Geometry check sheet. Reference: the model listing, model coordinates, mm. A direction names the side the tool comes from. Give positions to 0.01 mm unless a question says otherwise; leave off trailing zeros. Loops run counter-clockwise (first coordinate to the right, second up) from the corner with the lowest first, then second, coordinate; pieces in that order, holes last. Notation, with made-up numbers: (52, -37) -> (110, -37) arc R25 ccw to (110, -14) -> close; hole circle Ø11 at (7, 17.25). An arc over 180 degrees is marked (long way). Answer in a Markdown table with one row per item. Add a question column.
Autodesk Inventor part; units mm, degrees
ref_plane "YZ Plane" through (0, 0, 0) normal (1, 0, 0) x (0, 1, 0)
ref_plane "XZ Plane" through (0, 0, 0) normal (0, 1, 0) x (-1, 0, 0)
ref_plane "XY Plane" through (0, 0, 0) normal (0, 0, 1) x (1, 0, 0)
sketch "スケッチ1" plane through (0, 0, 0) normal (0, 0, 1) x (1, 0, 0)
  circle A0 centre (0, 0) radius 10
  circle A1 centre (0, 0) radius 2
  line L0 (0, -2) -> (0, -47)
  line L1 (10, 0) -> (10, -47)
  line L2 (10, -47) -> (-10, -47)
  line L3 (-10, -47) -> (-10, 0)
  circle A2 centre (0, -32) radius 1
  circle A3 centre (0, -42) radius 1
  circle A4 centre (0, -22) radius 1
  dimension "d1" = 4
  dimension "d0" = 20
  dimension "d2" = 45
  dimension "d9" = 2
  dimension "d10" = 2
  dimension "d11" = 2
  dimension "d31" = 10
  dimension "d32" = 22
extrude "押し出し1" add sketch "スケッチ1" along normal blind 2
sketch "スケッチ2" plane through (0, 0, 2) normal (0, 0, 1) x (1, 0, 0)
  circle A0 centre (0, -32) radius 1.7
  circle A1 centre (0, -22) radius 1.7
  circle A2 centre (0, -42) radius 1.7
  point P0 (0, 0)
  dimension "d12" = 3.4
  dimension "d13" = 3.4
  dimension "d14" = 3.4
extrude "押し出し2" cut sketch "スケッチ2" against normal blind 10
sketch "スケッチ3" plane through (0, 0, 0) normal (0, 0, -1) x (-1, 0, 0)
  line L0 (10, -47) -> (-10, -47)
  line L1 (10, -47) -> (5, -47)
  circle A0 centre (0, 0) radius 10
  line L2 (5, -47) -> (5, -8.6603)
  line L3 (10, 0) -> (10, -47)
  line L4 (10, -47) -> (10, 0)
  line L5 (-10, -47) -> (-10, 0)
  line L6 (-10, 0) -> (-10, -47)
  line L7 (-10, -47) -> (-5, -47)
  line L8 (-5, -47) -> (-5, -8.6603)
  dimension "d17" = 5
  dimension "d18" = 5
extrude "押し出し3" cut sketch "スケッチ3" against normal blind 10 contours L0 L2 A0 L3 | L0 L5 A0 L8
sketch "スケッチ4" plane through (0, 0, 0) normal (0, 0, -1) x (-1, 0, 0)
  circle A0 centre (0, 0) radius 5.5
  circle A1 centre (0, -5.5) radius 1.25
  circle A2 centre (0, 5.5) radius 1.25
  dimension "d21" = 11
  dimension "d22" = 2.5
  dimension "d23" = 2.5
extrude "押し出し4" cut sketch "スケッチ4" against normal blind 10 contours A2 A0 | A0 A2 | A1 A0 | A0 A1
fillet "フィレット1" radius 2 2 edges at (5, -8.6603, 1) (-5, -8.6603, 1)
properties part number "cutter_board"
1. Material ranges on L1, parallel to X at y = 0, z = 0.85; L2, parallel to X at y = -1.5, z = 1.8; L3, parallel to X at y = -16.5, z = 0.4, recorded low to high. Write a range as from..to.
2. Sectioned sample at B-B (y = -32). Enter the section's corners in (x, z), plus the area to 3 significant figures.
3. Sectioned sample at D-D (x = -8). Enter the section's corners in (y, z).
4. Sectioned sample at A-A (x = 0). Enter the section's corners in (y, z).
5. Sectioned sample at C-C (y = 0). Enter the section's corners in (x, z), plus the area to 3 significant figures.
6. Access from +Z, -Z, +X, -X, +Y, -Y to the whole of each face (thin tool, end or side, straight path). Record for faces 5 (the face through (0.27, -6.72, 0.99)), 6 (the face through (5, -29, 1)).
7. Release check for a two-part mould opening along Y. For faces 1 (the face through (-5.227, -8.822, 0.986)), 2 (the face through (-5, -29, 1)), 3 (the face through (0, 10, 1)), 4 (the face through (-0.37, -43.66, 1.01)) record: released by +Y, released by -Y, zero draft, split by the parting line, or undercut.
8. Gauge pin test, flat ends, axial feed: pin 1 Ø0.6 at (y, z) = (-25.5, 1.5) entering from +X; pin 2 Ø3 at (x, y) = (0, -5.5) entering from -Z. Record the tip position at first contact, or that the pin passes through.
Response:
| question | item | result |
|---|---|---|
| 1 | L1 | x = -10..-2, 2..10 |
| 1 | L2 | x = -9.89..-1.32, 1.32..9.89 |
| 1 | L3 | x = -5..5 |
| 2 | outline | (-5, 0) -> (-1.7, 0) -> (-1.7, 2) -> (-5, 2) -> close; (1.7, 0) -> (5, 0) -> (5, 2) -> (1.7, 2) -> close |
| 2 | area | 13.2 mm2 |
| 3 | outline | (-6, 0) -> (6, 0) -> (6, 2) -> (-6, 2) -> close |
| 4 | outline | (-47, 0) -> (-43.7, 0) -> (-43.7, 2) -> (-47, 2) -> close; (-40.3, 0) -> (-33.7, 0) -> (-33.7, 2) -> (-40.3, 2) -> close; (-30.3, 0) -> (-23.7, 0) -> (-23.7, 2) -> (-30.3, 2) -> close; (-20.3, 0) -> (-6.75, 0) -> (-6.75, 2) -> (-20.3, 2) -> close; (-4.25, 0) -> (-2, 0) -> (-2, 2) -> (-4.25, 2) -> close; (2, 0) -> (4.25, 0) -> (4.25, 2) -> (2, 2) -> close; (6.75, 0) -> (10, 0) -> (10, 2) -> (6.75, 2) -> close |
| 5 | outline | (-10, 0) -> (-2, 0) -> (-2, 2) -> (-10, 2) -> close; (2, 0) -> (10, 0) -> (10, 2) -> (2, 2) -> close |
| 5 | area | 32.0 mm2 |
| 6 | face 5 | +Z, -Z |
| 6 | face 6 | +Z, -Z, +X, -Y |
| 7 | face 1 | released by -Y |
| 7 | face 2 | zero draft |
| 7 | face 3 | split by the parting line |
| 7 | face 4 | undercut |
| 8 | pin 1 | stops at x = 5 |
| 8 | pin 2 | stops at z = 0 |
